from build123d import *

# Parameters (mm, degrees)
F0_W     = 48
F0_H     = 48
F1_DEPTH = 48
F3_DEPTH = 48
F4_SIZE  = 1


with BuildPart() as f1:
    # F0 (on Front) → F1 (new body)
    with BuildSketch(Plane.XZ):
        Rectangle(F0_W, F0_H)
    extrude(amount=F1_DEPTH)

    # F2 (on face) → F3 (cut)
    with BuildSketch(Plane.XZ.offset(48)):
        with BuildLine():
            ThreePointArc((-9, 24), (0, 15), (9, 24))
            Line((9, 24), (-9, 24))
        make_face()
    extrude(amount=-F3_DEPTH, mode=Mode.SUBTRACT)

    # F4
    f4_edges = [f1.edges().sort_by_distance(p)[0] for p in [
        (16.5, -48, 24),
        (-16.5, -48, 24),
        (24, -24, 24),
        (16.5, 0, 24),
        (-16.5, 0, 24),
        (-24, -24, 24),
    ]]
    chamfer(f4_edges, length=F4_SIZE)


solid = f1.part
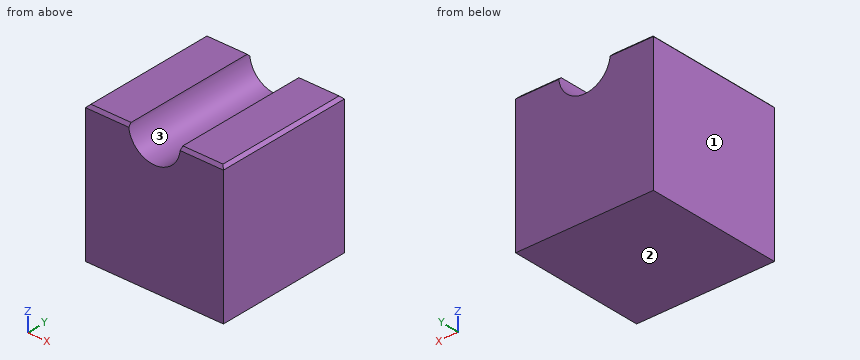
Build history of the part. All positions in model axes, mm. Face numbers are marked on the shaded views. Give positions to 0.01 mm unless a question says otherwise; leave off trailing zeros. Order: outer loops, then holes, each group sorted by start corner. A loop starts at its lowest first (then second) coordinate and runs counter-clockwise, first axis right, second up. Notation, with made-up numbers: M 89.25,76 L 98.25,76 A35 cw 98.25,109 Z; hole C 8.25,40.25 d1. An arc over 180 degrees is marked long. Put each result on its own line as item: value.
Item 1: Wall check: probe 1 along X at (y, z) = (-34, 18); probe 2 along X at (y, z) = (-9, 16); probe 3 along Z at (x, y) = (8, -5.5). Give the ranges that are in metal, low to high.
Results are:
probe 1: -24 to -6.71, 6.71 to 24
probe 2: -24 to -4.12, 4.12 to 24
probe 3: -24 to 19.88
Item 2: Drop flat-ended pins along their axis: pin 1 Ø6 at (x, z) = (-0.5, 18.5) entering from -Y; pin 2 Ø1.5 at (x, z) = (-6.5, 10) entering from +Y. Give the stop position or say it passes through.
Results are:
pin 1: through
pin 2: y = 0
Item 3: Pull direction X, two halves, no side cores. Call the marked faces 1, 2 and 3: +X half, -X half, draft (parallel to the pull), parting line (faces both ways), or undercut.
Results are:
face 1: -X half
face 2: draft
face 3: undercut
Item 4: Cut at A-A on y = -42.5. Write the cut outline in (x, z).
Results are:
outline: M -24,-24 L 24,-24 L 24,23 L 23,24 L 9,24 A9 cw -9,24 L -23,24 L -24,23 Z
Item 5: Cut at B-B on x = 0. Write the cut outline in (y, z).
Results are:
outline: M -48,-24 L 0,-24 L 0,15 L -48,15 Z
